Design review of the part built by this model. Coordinates are the model's own, in mm. Coordinates: 2 decimals unless noted, no trailing zeros. Write each loop counter-clockwise with the first axis right and the second up, starting at its lowest first coordinate (ties: lowest second). Pieces come first, ordered by that corner, then holes.
Q1. For L1, parallel to Y at x = 63.2, z = 1.1; L2, parallel to X at y = -8.5, z = 1.1; L3, parallel to X at y = -4.75, z = 0.2, list the stretches that pass through material, from the lowest coordinate up.
Q2. Take a section at C-C, the plane z = 0.6. Write out the cut boundary in (x, y), plus the area to 3 significant figures.
Q3. For pin 1 Ø7.5 at (x, y) = (-62.8, -7.5) entering from -Z; pin 2 Ø1 at (y, z) = (-2, 0.5) entering from -X, all flat-tipped, find the tip position at first contact; note any pin that passes through.
Q4. Take a section at A-A, the plane x = 0.2. Write out the cut boundary in (y, z), plus the area to 3 significant figures.
Q5. Take a section at B-B, the plane y = -7.5. Write out the cut boundary in (x, z), plus the area to 3 significant figures.
from build123d import *

# Parameters (mm, degrees)
F1_DEPTH = 2
F3_DEPTH = 12.5


with BuildPart() as f1:
    # F0 (on Top) → F1 (new body)
    with BuildSketch(Plane.XY):
        with BuildLine():
            Line((67.5, 0), (-67.5, 0))
            ThreePointArc((-67.5, 0), (-71.0355339059, -1.4644660941), (-72.5, -5))
            Line((-72.5, -5), (-72.5, -10))
            ThreePointArc((-72.5, -10), (-71.0355339059, -13.5355339059), (-67.5, -15))
            Line((-67.5, -15), (67.5, -15))
            ThreePointArc((67.5, -15), (71.0355339059, -13.5355339059), (72.5, -10))
            Line((72.5, -10), (72.5, -5))
            ThreePointArc((72.5, -5), (71.0355339059, -1.4644660941), (67.5, 0))
        make_face()
    extrude(amount=F1_DEPTH)

    # F2 (on face) → F3 (cut, symmetric)
    with BuildSketch(Plane.XY.offset(2)):
        with BuildLine():
            Line((-62.8, -7.5), (-65.1, -7.5))
            ThreePointArc((-65.1, -7.5), (-62.8, -9.8), (-60.5, -7.5))
            Line((-60.5, -7.5), (-62.8, -7.5))
        make_face()
        with BuildLine():
            ThreePointArc((-60.5, -7.5), (-62.8, -5.2), (-65.1, -7.5))
            Line((-65.1, -7.5), (-62.8, -7.5))
            Line((-62.8, -7.5), (-60.5, -7.5))
        make_face()
        with BuildLine():
            ThreePointArc((2.5, -7.5), (0.2, -5.2), (-2.1, -7.5))
            Line((-2.1, -7.5), (0.2, -7.5))
            Line((0.2, -7.5), (2.5, -7.5))
        make_face()
        with BuildLine():
            Line((0.2, -7.5), (-2.1, -7.5))
            ThreePointArc((-2.1, -7.5), (0.2, -9.8), (2.5, -7.5))
            Line((2.5, -7.5), (0.2, -7.5))
        make_face()
        with BuildLine():
            ThreePointArc((65.5, -7.5), (63.2, -5.2), (60.9, -7.5))
            ThreePointArc((60.9, -7.5), (63.2, -9.8), (65.5, -7.5))
        make_face()
    extrude(amount=F3_DEPTH, both=True, mode=Mode.SUBTRACT)


solid = f1.part
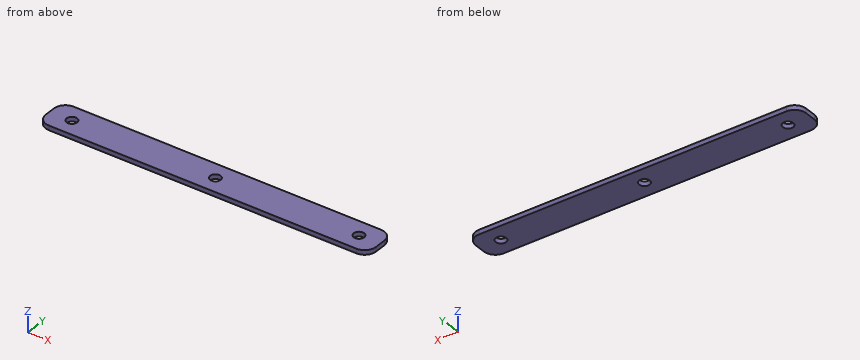
Responses:
1. L1: y = -15 to -9.8, -5.2 to 0
1. L2: x = -72.5 to -64.87, -60.73 to -1.87, 2.27 to 61.13, 65.27 to 72.5
1. L3: x = -72.49 to 72.49
2. outline: (-72.5, -10) arc R5 ccw to (-67.5, -15) - (67.5, -15) arc R5 ccw to (72.5, -10) - (72.5, -5) arc R5 ccw to (67.5, 0) - (-67.5, 0) arc R5 ccw to (-72.5, -5) - close; hole circle Ø4.6 at (-62.8, -7.5); hole circle Ø4.6 at (0.2, -7.5); hole circle Ø4.6 at (63.2, -7.5)
2. area: 2,100 mm2
3. pin 1: stops at z = 0
3. pin 2: stops at x = -71.83
4. outline: (-15, 0) - (-9.8, 0) - (-9.8, 2) - (-15, 2) - close; (-5.2, 0) - (0, 0) - (0, 2) - (-5.2, 2) - close
4. area: 20.8 mm2
5. outline: (-72.5, 0) - (-65.1, 0) - (-65.1, 2) - (-72.5, 2) - close; (-60.5, 0) - (-2.1, 0) - (-2.1, 2) - (-60.5, 2) - close; (2.5, 0) - (60.9, 0) - (60.9, 2) - (2.5, 2) - close; (65.5, 0) - (72.5, 0) - (72.5, 2) - (65.5, 2) - close
5. area: 262 mm2
